Here's how the part is built. I have some questions about the finished solid (model axes, mm). A direction names the side the tool comes from. Round coordinates to 2 decimals unless told otherwise and drop trailing zeros. Order: outer loops, then holes, each group sorted by start corner. A loop starts at its lowest first (then second) coordinate and runs counter-clockwise, first axis right, second up. Notation, with made-up numbers: (-4.75, 25) -> (21.25, 25) arc R31 cw to (21.25, 54) -> close; hole circle Ø8 at (-13.5, 44). An arc over 180 degrees is marked (long way). Use a Markdown table: item, result. Add a question column.
from build123d import *

# Parameters (mm, degrees)
BOSS_EXTRUDE1_DEPTH = 25.4
SKETCH2_R           = 4.7625
CUT_EXTRUDE1_DEPTH  = 25.4
SKETCH3_R           = 4.7625
CUT_EXTRUDE2_DEPTH  = 16.875


with BuildPart() as part:
    # Sketch1 → Boss-Extrude1 (new body)
    with BuildSketch(Plane(origin=(0, 0, 0), x_dir=(0, 0, -1), z_dir=(1, 0, 0))):
        Polygon((0, 0), (-25.4, 0), (-25.4, 3.175), (-1.315128061, 3.175), (15.715448212, 20.205576272), (17.960512242, 17.960512242), align=None)
    extrude(amount=BOSS_EXTRUDE1_DEPTH)

    # Sketch2 → Cut-Extrude1 (cut)
    with BuildSketch(Plane(origin=(0, 3.175, 0), x_dir=(1, 0, 0), z_dir=(0, 1, 0))):
        with Locations((12.7, -12.7)):
            Circle(SKETCH2_R)
    extrude(amount=-CUT_EXTRUDE1_DEPTH, mode=Mode.SUBTRACT)

    # Sketch3 → Cut-Extrude2 (cut, through all)
    with BuildSketch(Plane(origin=(0, 2.24506403, 2.24506403), x_dir=(1, 0, 0), z_dir=(0, 0.707106781, 0.707106781))):
        with Locations((12.7, 12.7)):
            Circle(SKETCH3_R)
    extrude(amount=-CUT_EXTRUDE2_DEPTH, mode=Mode.SUBTRACT)


solid = part.part
(1) I want a section at D-D on x = 16.25. List the corners of the cut face in (y, z) for me (3 decimals), and give its area (3 significant figures).
(2) If we mould it in two halves opening along X, with no side actions, what happens to faces 1 (the cylindrical face through (7.942, 1.61, 12.491)), 2 (the flat face through (0, 3, 0)), 3 (the flat face through (12.52, 15.36, -10.87))? For each: pulls with the +X half, pulls with the -X half, needs draft (parallel to the pull), parting line crosses it, or undercut.
(3) I'm going to push flat-ended pins straight in: P1, Ø15, axis at x = 12.7, z = 12.7, coming from the +Y side (3 decimals); P2, Ø8, axis at x = 9, y = 4.5, coming from the -Z side; P3, Ø10, axis at y = 14.5, z = -8, coming from the -X side; P4, Ø4, axis at x = 13, y = 9.5, coming from the +Z side. Where does each tip first touch, or does it pass through?
(4) I want a section at B-B on x = 8.5. List the corners of the cut face in (y, z) for me (3 decimals).
(5) Please list where these lines run through material, in increasing order: probe 1 along X at (y, z) = (0.85, 12.7); probe 2 along Y at (x, z) = (7, 4) (3 decimals); probe 3 along X at (y, z) = (2.75, 9.5). Write a range as from..to.
(6) I want a section at A-A on z = 12.7. List the corners of the cut face in (x, y) for me (1 decimal), and give its area (3 significant figures).
(7) On a 3-axis mill with a long thin cutter (end or side, diameter ignored), from which of +Z, -Z, +X, -X, +Y, -Y can I reach the whole of each face in a straight line? I mean faces 4 (the flat face through (13, 3.175, 19)), 5 (the flat face through (13, 13, -13)). Say none if no direction works.
Output:
| question | item | result |
|---|---|---|
| 1 | outline | (0, 0) -> (6.735, -6.735) -> (8.98, -4.49) -> (3.175, 1.315) -> (3.175, 9.525) -> (0, 9.525) -> close; (0, 15.875) -> (3.175, 15.875) -> (3.175, 25.4) -> (0, 25.4) -> close; (11.225, -11.225) -> (17.961, -17.961) -> (20.206, -15.715) -> (13.47, -8.98) -> close |
| 1 | area | 117 mm² |
| 2 | face 1 | undercut |
| 2 | face 2 | pulls with the -X half |
| 2 | face 3 | needs draft |
| 3 | P1 | y = 3.175 |
| 3 | P2 | z = -8.38 |
| 3 | P3 | x = 0 |
| 3 | P4 | z = -3.01 |
| 4 | outline | (0, 0) -> (7.393, -7.393) -> (9.638, -5.148) -> (3.175, 1.315) -> (3.175, 10.455) -> (0, 10.455) -> close; (0, 14.945) -> (3.175, 14.945) -> (3.175, 25.4) -> (0, 25.4) -> close; (10.568, -10.568) -> (17.961, -17.961) -> (20.206, -15.715) -> (12.813, -8.323) -> close |
| 5 | probe 1 | 0..7.94, 17.46..25.4 |
| 5 | probe 2 | 0..3.175 |
| 5 | probe 3 | 0..9.17, 16.23..25.4 |
| 6 | outline | (0, 0) -> (7.9, 0) -> (7.9, 3.2) -> (0, 3.2) -> close; (17.5, 0) -> (25.4, 0) -> (25.4, 3.2) -> (17.5, 3.2) -> close |
| 6 | area | 50.4 mm² |
| 7 | face 4 | +Z, +X, -X, +Y |
| 7 | face 5 | -Z, +X, -X, -Y |
